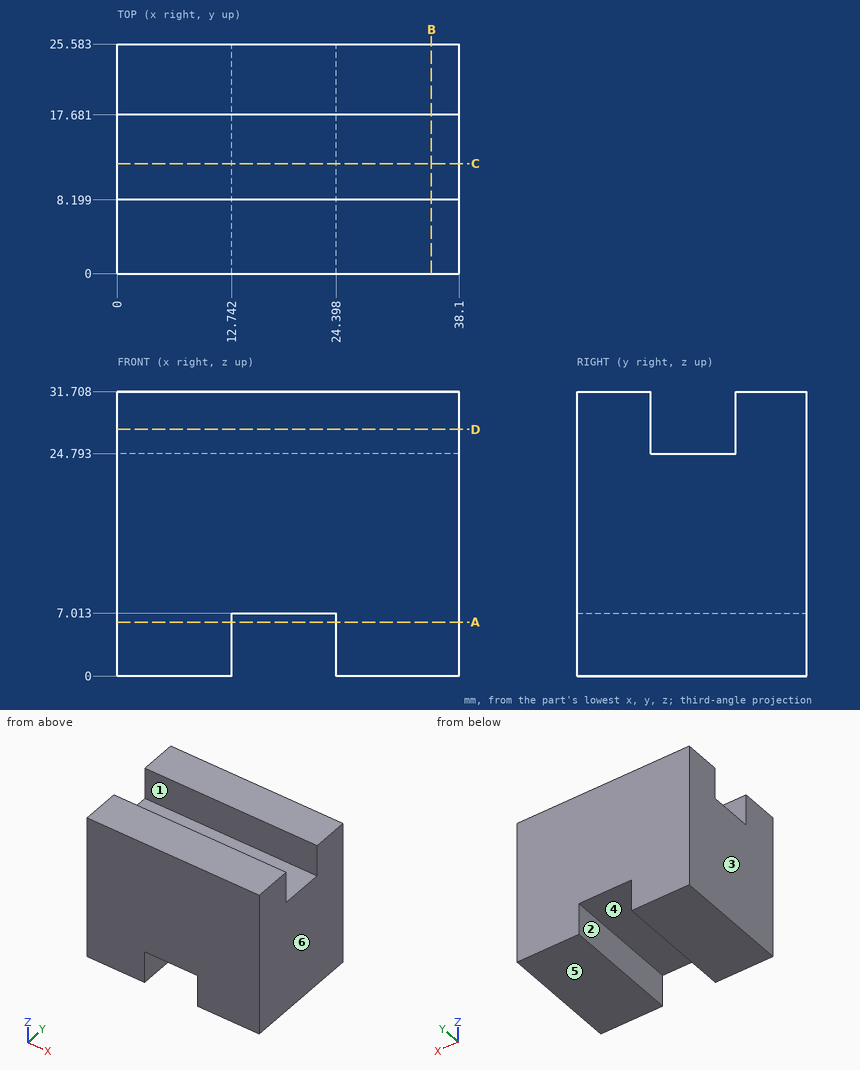
The drawing under review shows one solid part. Ordinate dimensions are in mm from its lowest x, y, z. A direction names the side the tool comes from. Coordinates: 2 decimals unless noted, no trailing zeros. Write each loop counter-clockwise with the first axis right and the second up, starting at its lowest first coordinate (ties: lowest second). Pieces come first, ordered by that corner, then holes. Notation, with made-up numbers: M 51.5,19.5 L 99.5,19.5 A18 ccw 99.5,48.5 Z; hole C 12,-11 d6. An arc over 180 degrees is marked long. Put each result on its own line as item: value.
1) Clearance check with a flat-ended pin moving along its axis: pin 1 Ø3 at (x, y) = (24.5, 13.5) entering from +Z. State where the tip first meets the part, or that it passes through.
Computed:
pin 1: stops at z = 24.79
2) Add section D-D on z = 27.5. Give the boundary of the cut face in (x, y).
Computed:
outline: M 0,0 L 38.1,0 L 38.1,8.2 L 0,8.2 Z; M 0,17.68 L 38.1,17.68 L 38.1,25.58 L 0,25.58 Z
3) Wall thickness on probe 1 along X at (y, z) = (13.75, 2); probe 2 along Z at (x, y) = (18.5, 20.5); probe 3 along Z at (x, y) = (11.5, 14): over which ranges is each line inside the solid? List them lowest first. Write a range as [from, to].
Computed:
probe 1: x = [0, 12.74], [24.4, 38.1]
probe 2: z = [7.01, 31.71]
probe 3: z = [0, 24.79]
4) Add section B-B on x = 35. Give the boundary of the cut face in (y, z).
Computed:
outline: M 0,0 L 25.58,0 L 25.58,31.71 L 17.68,31.71 L 17.68,24.79 L 8.2,24.79 L 8.2,31.71 L 0,31.71 Z
5) For the marked faces 1, 2 and 3, list the 3-axis set-ups (+Z, -Z, +X, -X, +Y, -Y) from which the entire face can be reached by the end or side of a thin tool; tool diameter is ignored.
Computed:
face 1: +Z, +X, -X
face 2: -Z, +Y, -Y
face 3: +Z, -Z, -X, +Y, -Y
6) Add section A-A on z = 6. Give the boundary of the cut face in (x, y).
Computed:
outline: M 0,0 L 12.74,0 L 12.74,25.58 L 0,25.58 Z; M 24.4,0 L 38.1,0 L 38.1,25.58 L 24.4,25.58 Z
7) Draft analysis for pull direction X (two halves, no side actions). For the marked faces 4, 5 and 6, state which applies: released by +X, released by -X, zero draft, split by the parting line, or undercut.
Computed:
face 4: undercut
face 5: zero draft
face 6: released by +X
8) Add section C-C on y = 12.25. Give the boundary of the cut face in (x, z).
Computed:
outline: M 0,0 L 12.74,0 L 12.74,7.01 L 24.4,7.01 L 24.4,0 L 38.1,0 L 38.1,24.79 L 0,24.79 Z
